Read the model definition and answer for the solid it produces. Units are mm, in the model's axes. Face numbers are marked on the shaded views. A direction names the side the tool comes from. Coordinates: 2 decimals unless noted, no trailing zeros. Order: outer loops, then holes, each group sorted by start corner. A loop starts at its lowest first (then second) coordinate and runs counter-clockwise, first axis right, second up.
```python
from build123d import *
from build123d.topology import SkipClean

# Parameters (mm, degrees)
SKETCH_1_R      = 7.5
EXTRUDE_1_DEPTH = 10
SKETCH_2_R      = 10
EXTRUDE_2_DEPTH = 3
SKETCH_3_R      = 7.5
EXTRUDE_3_DEPTH = 5
EXTRUDE_START   = 5
EXTRUDE_4_DEPTH = 5


with BuildPart() as part:
    # 草图1 → 凸台-拉伸1 (new body)
    with BuildSketch(Plane(origin=(0, 0, 0), x_dir=(1, 0, 0), z_dir=(0, 1, 0))):
        with Locations(Location((0, 0, 0), (0, 0, 270))):
            Circle(SKETCH_1_R)
    extrude(amount=EXTRUDE_1_DEPTH)

    # 草图2 → 凸台-拉伸2 (add)
    with BuildSketch(Plane(origin=(0, 10, 0), x_dir=(1, 0, 0), z_dir=(0, 1, 0))):
        with Locations(Location((0, 0, 0), (0, 0, 270))):
            Circle(SKETCH_2_R)
    extrude(amount=EXTRUDE_2_DEPTH)

    # 草图3 → 凸台-拉伸3 (add)
    with BuildSketch(Plane(origin=(0, 13, 0), x_dir=(1, 0, 0), z_dir=(0, 1, 0))):
        with Locations(Location((0, 0, 0), (0, 0, 270))):
            Circle(SKETCH_3_R)
    extrude(amount=EXTRUDE_3_DEPTH)

    # 草图4 → 凸台-拉伸4 (add)
    with SkipClean():  # the faces are left unmerged after this step: merging them gives an invalid solid
        with BuildSketch(Plane.XZ.offset(EXTRUDE_START)):
            with BuildLine():
                Line((-1.048132204, 7.426400129), (-1.048132204, -7.426400129))
                ThreePointArc((-1.048132204, -7.426400129), (0, -7.5), (1.048132204, -7.426400129))
                Line((1.048132204, -7.426400129), (1.048132204, 7.426400129))
                ThreePointArc((1.048132204, 7.426400129), (0, 7.5), (-1.048132204, 7.426400129))
            make_face()
        extrude(amount=-EXTRUDE_4_DEPTH)


solid = part.part
```
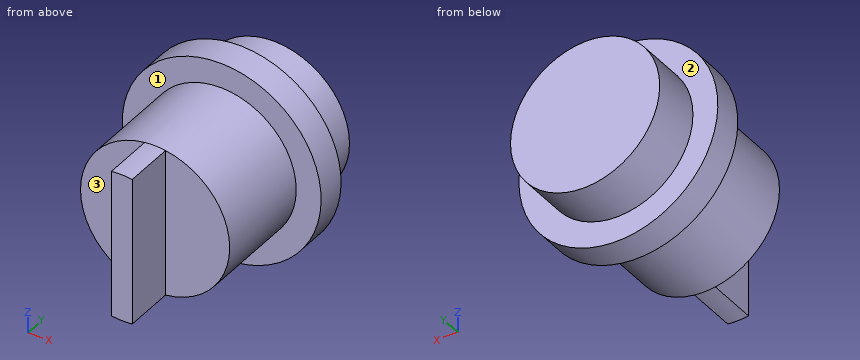
1) A cutting plane is placed at A-A, the plane z = 0. Determine the outline of the cut face in (x, y), and give its area (3 significant figures).
A:
outline: (-10, 10) - (-7.5, 10) - (-7.5, 0) - (-1.05, 0) - (-1.05, -5) - (1.05, -5) - (1.05, 0) - (7.5, 0) - (7.5, 10) - (10, 10) - (10, 13) - (7.5, 13) - (7.5, 18) - (-7.5, 18) - (-7.5, 13) - (-10, 13) - close
area: 295 mm2
2) Which of the six approach directions +Z, -Z, +X, -X, +Y, -Y give full straight-line access (tool end or side, diameter ignored) to the marked faces 1, 2 and 3?
A:
face 1: -Y
face 2: +Y
face 3: +Z, -Z, -X, -Y
3) A cutting plane is placed at C-C, the plane y = 2.25. Determine the outline of the cut face in (x, z).
A:
outline: circle Ø15 at (0, 0)
4) Straight lines are drawn through the part: line 1 (Y direction, x = -5.25, z = 4.25); line 2 (Z direction, x = -0.25, y = -1); line 3 (Y direction, x = 0.75, z = -9). For each, find the intervals that lie inside material, in ascending order.
A:
line 1: y = 0 to 18
line 2: z = -7.5 to 7.5
line 3: y = 10 to 13
5) A cutting plane is placed at D-D, the plane z = 5.25. Determine the outline of the cut face in (x, y), and give its area (3 significant figures).
A:
outline: (-8.51, 10) - (-5.36, 10) - (-5.36, 0) - (-1.05, 0) - (-1.05, -5) - (1.05, -5) - (1.05, 0) - (5.36, 0) - (5.36, 10) - (8.51, 10) - (8.51, 13) - (5.36, 13) - (5.36, 18) - (-5.36, 18) - (-5.36, 13) - (-8.51, 13) - close
area: 222 mm2
6) Flat-ended cylindrical pins translate along their axes: pin 1 Ø1.9 at (x, z) = (-3.5, 1) entering from -Y; pin 2 Ø6 at (x, y) = (-1, 0) entering from +Z; pin 3 Ø3 at (y, z) = (1, 3) entering from -X. Find the tip coordinate at first contact, or state that the pin passes through.
A:
pin 1: stops at y = 0
pin 2: stops at z = 7.5
pin 3: stops at x = -7.35
7) A cutting plane is placed at B-B, the plane x = 0. Determine the outline of the cut face in (y, z).
A:
outline: (-5, -7.5) - (10, -7.5) - (10, -10) - (13, -10) - (13, -7.5) - (18, -7.5) - (18, 7.5) - (13, 7.5) - (13, 10) - (10, 10) - (10, 7.5) - (-5, 7.5) - close
